Geometry check sheet. Reference: the model listing, model coordinates, mm. A direction names the side the tool comes from. Round coordinates to 2 decimals unless told otherwise and drop trailing zeros. Order: outer loops, then holes, each group sorted by start corner. A loop starts at its lowest first (then second) coordinate and runs counter-clockwise, first axis right, second up.
(1) Material ranges on line 1 along X through (y, z) = (-5.4, 0); line 2 along Y through (x, z) = (-5, -0.75); line 3 along Y through (x, z) = (5, -0.75), recorded low to high.
(2) Sectioned sample at A-A (x = -2.25). Record the boundary of the cut face in (y, z), plus the area to 3 significant figures.
(3) Set-up check for faces 1 (the face through (3.8, -0.1, -2.5)), 2 (the face through (28.5, 0, 0)): record each of +Z, -Z, +X, -X, +Y, -Y from which the full face is reachable in a straight line by a thin tool's end or side.
(4) Sectioned sample at C-C (y = 5.25). Record the boundary of the cut face in (x, z).
(5) Sectioned sample at B-B (z = -3.5). Record the boundary of the cut face in (x, y).
(6) Go/stop test with flat-tipped pins: pin 1 (3 mm diameter, centred on y = 2, z = 0, fed in from -X); pin 2 (4 mm diameter, centred on x = 13, z = -0.5, fed in from +Y); pin 3 (3.5 mm diameter, centred on x = -2.25, z = 0, fed in from -Y); pin 4 (1.5 mm diameter, centred on y = -4.5, z = 1.5, fed in from +X). Record where each tip stops, or that it passes through.
(7) Sectioned sample at D-D (z = 0). Give the number of separate pieces and of enclosed holes in the cut face, plus the area to 3 significant figures.
from build123d import *

# Parameters (mm, degrees)
BASEHEAD_DEPTH      = 3.5
THDSCHPAT_COUNT     = 30
THDSCHPAT_PITCH     = 0.8
BOSS_EXTRUDE1_DEPTH = 5
SKETCH3_R           = 2
CUT_EXTRUDE1_DEPTH  = 17


with BuildPart() as part:
    # BaseHeadSke → BaseHead (new body)
    with BuildSketch(Plane(origin=(0, 0, 0), x_dir=(0, 0, -1), z_dir=(1, 0, 0))):
        Polygon((0, 4.618802154), (-4, 2.309401077), (-4, -2.309401077), (0, -4.618802154), (4, -2.309401077), (4, 2.309401077), align=None)
    extrude(amount=BASEHEAD_DEPTH)

    # HeadChamferSke → HeadChamfer (revolve, cut)
    with BuildSketch(Plane.XY):
        Polygon((0, 4.618802154), (0, 4), (0.35726559, 4.618802154), align=None)
    revolve(axis=Axis((0, 0, 0), (1, 0, 0)), mode=Mode.SUBTRACT)

    # BodySke → BaseBody (revolve)
    with BuildSketch(Plane.XY, mode=Mode.PRIVATE) as basebody_sk:
        Polygon((0, 0), (0, 2.5), (28.055, 2.5), (28.5, 2.055), (28.5, 0), align=None)
    revolve(basebody_sk.sketch.rotate(Axis((0, 0, 0), (1, 0, 0)), 90), axis=Axis((0, 0, 0), (1, 0, 0)))

    # ThdSchSke → ThreadSchematic (revolve, cut)
    with BuildSketch(Plane.XY, mode=Mode.PRIVATE) as threadschematic_sk:
        Polygon((27.255, 3.01384174), (27.255, 2.5), (27.51192087, 2.055), (27.76884174, 2.5), (27.76884174, 3.01384174), align=None)
    threadschematic = revolve(threadschematic_sk.sketch.rotate(Axis((0, 0, 0), (1, 0, 0)), 90), axis=Axis((0, 0, 0), (1, 0, 0)), mode=Mode.SUBTRACT)

    # ThdSchPat: ThreadSchematic ×30
    with Locations(*[(-i * THDSCHPAT_PITCH, 0, 0) for i in range(1, THDSCHPAT_COUNT)]):
        add(threadschematic, mode=Mode.SUBTRACT)

    # Sketch1 → Boss-Extrude1 (add, symmetric)
    with BuildSketch(Plane.XY):
        Polygon((-8, 7.5), (3.5, 7.5), (3.5, -7.5), (-8, -7.5), (-8, -4.608070982), (0, -4.608070982), (0, 4.608070982), (-8, 4.608070982), align=None)
    extrude(amount=BOSS_EXTRUDE1_DEPTH, both=True)

    # Sketch3 → Cut-Extrude1 (cut)
    with BuildSketch(Plane.XZ.offset(7.5)):
        with Locations(Location((-2.25, 0, 0), (0, 0, 270))):
            Circle(SKETCH3_R)
    extrude(amount=-CUT_EXTRUDE1_DEPTH, mode=Mode.SUBTRACT)


solid = part.part
Answer below:
1. line 1: x = -8 to -4.25, -0.25 to 3.5
1. line 2: y = -7.5 to -4.61, 4.61 to 7.5
1. line 3: y = -2.12 to 2.12
2. outline: (-7.5, -5) - (-4.61, -5) - (-4.61, -2) - (-7.5, -2) - close; (-7.5, 2) - (-4.61, 2) - (-4.61, 5) - (-7.5, 5) - close; (4.61, -5) - (7.5, -5) - (7.5, -2) - (4.61, -2) - close; (4.61, 2) - (7.5, 2) - (7.5, 5) - (4.61, 5) - close
2. area: 34.7 mm2
3. face 1: +X
3. face 2: +Z, -Z, +X, +Y, -Y
4. outline: (-8, -5) - (3.5, -5) - (3.5, 5) - (-8, 5) - close; hole circle Ø4 at (-2.25, 0)
5. outline: (-8, -7.5) - (3.5, -7.5) - (3.5, 7.5) - (-8, 7.5) - (-8, 4.61) - (0, 4.61) - (0, -4.61) - (-8, -4.61) - close
6. pin 1: stops at x = 0
6. pin 2: stops at y = 2.5
6. pin 3: passes through
6. pin 4: stops at x = 3.5
7. separate pieces: 3
7. enclosed holes: 0
7. area: 194 mm2
